Check sheet for the modelled part. Datum: model origin and axes. Units: mm. A direction names the side the tool comes from. Round coordinates to 2 decimals unless told otherwise and drop trailing zeros. Write each loop counter-clockwise with the first axis right and the second up, starting at its lowest first coordinate (ties: lowest second). Pieces come first, ordered by that corner, then holes.
Item 1: Tool access check on faces 1 (the cylindrical face through (-10.006, 18.725, -1.037)), 2 (the cylindrical face through (16.116, 4.93, 0.914)). Record the directions out of +Z, -Z, +X, -X, +Y, -Y that give a thin tool (end or side, any length) a straight path to the whole face; none if there is none.
Item 2: Material ranges on line 1 (X direction, y = 5.5, z = 0); line 2 (X direction, y = 14.75, z = 0); line 3 (Z direction, x = 12, y = 4.5), recorded low to high.
Item 3: Cross-section at C-C on y = 21.75. Enter the section's corners in (x, z), plus the area to 3 significant figures.
Item 4: Cross-section at A-A on z = 0. Enter the section's corners in (x, y).
Item 5: Cross-section at D-D on y = 2.25. Enter the section's corners in (x, z).
Item 6: Go/stop test with flat-tipped pins: pin 1 Ø5 at (x, y) = (4.5, 20.5) entering from +Z; pin 2 Ø3.5 at (x, z) = (-12, 0) entering from +Y; pin 3 Ø12 at (x, y) = (-12, 19.5) entering from -Z; pin 4 Ø1 at (y, z) = (15.5, 6) entering from +X. Record where each tip stops, or that it passes through.
Item 7: Cross-section at B-B on x = -12. Enter the section's corners in (y, z), plus the area to 3 significant figures.
Item 8: Release check for a two-part mould opening along Z. For faces 3 (the cylindrical face through (-19.334, 12.818, 2.539)), 4 (the cylindrical face through (-7.884, 4.93, 0.914)), 5 (the flat face through (0, 0, 0)) record: +Z half, -Z half, draft (parallel to the pull), parting line (faces both ways), or undercut.
from build123d import *

# Parameters (mm, degrees)
SKETCH1_R                                 = 19.5
BOSS_EXTRUDE1_DEPTH                       = 26
CSK_FOR_8_FLAT_HEAD_MACHINE_SCREW_2_COUNT = 2
CSK_FOR_8_FLAT_HEAD_MACHINE_SCREW_2_PITCH = 24


with BuildPart() as part:
    # Sketch1 → Boss-Extrude1 (new body)
    with BuildSketch(Plane(origin=(0, 0, 0), x_dir=(1, 0, 0), z_dir=(0, 1, 0))):
        with Locations(Location((0, 0, 0), (0, 0, 90))):
            Circle(SKETCH1_R)
    extrude(amount=BOSS_EXTRUDE1_DEPTH)

    # Sketch3 → CSK for #8 Flat Head Machine Screw (100)1 (revolve, cut)
    with BuildSketch(Plane(origin=(12, 0, 0), x_dir=(0, 0, -1), z_dir=(1, 0, 0))):
        Polygon((0, 0), (0, 26), (2.2479, 26), (2.2479, 11.651767624), (4.2164, 10), (4.2164, 0), align=None)
    csk_for_8_flat_head_machine_screw_100 = revolve(axis=Axis((12, -6.35, 0), (0, 1, 0)), mode=Mode.SUBTRACT)

    # CSK for _8 Flat Head Machine Screw _ 2: CSK for #8 Flat Head Machine Screw (100)1 ×2
    with Locations(*[(-i * CSK_FOR_8_FLAT_HEAD_MACHINE_SCREW_2_PITCH, 0, 0) for i in range(1, CSK_FOR_8_FLAT_HEAD_MACHINE_SCREW_2_COUNT)]):
        add(csk_for_8_flat_head_machine_screw_100, mode=Mode.SUBTRACT)


solid = part.part
Response values:
1. face 1: +Y, -Y
1. face 2: -Y
2. line 1: x = -19.5 to -16.22, -7.78 to 7.78, 16.22 to 19.5
2. line 2: x = -19.5 to -14.25, -9.75 to 9.75, 14.25 to 19.5
2. line 3: z = -15.37 to -4.22, 4.22 to 15.37
3. outline: circle Ø39 at (0, 0); hole circle Ø4.5 at (-12, 0); hole circle Ø4.5 at (12, 0)
3. area: 1,160 mm2
4. outline: (-19.5, 0) - (-16.22, 0) - (-16.22, 10) - (-14.25, 11.65) - (-14.25, 26) - (-19.5, 26) - close; (-9.75, 11.65) - (-7.78, 10) - (-7.78, 0) - (7.78, 0) - (7.78, 10) - (9.75, 11.65) - (9.75, 26) - (-9.75, 26) - close; (14.25, 11.65) - (16.22, 10) - (16.22, 0) - (19.5, 0) - (19.5, 26) - (14.25, 26) - close
5. outline: circle Ø39 at (0, 0); hole circle Ø8.43 at (-12, 0); hole circle Ø8.43 at (12, 0)
6. pin 1: stops at z = 19.4
6. pin 2: passes through
6. pin 3: stops at z = -18.55
6. pin 4: stops at x = 18.71
7. outline: (0, -15.37) - (26, -15.37) - (26, -2.25) - (11.65, -2.25) - (10, -4.22) - (0, -4.22) - close; (0, 4.22) - (10, 4.22) - (11.65, 2.25) - (26, 2.25) - (26, 15.37) - (0, 15.37) - close
7. area: 640 mm2
8. face 3: parting line
8. face 4: undercut
8. face 5: draft
